from build123d import *

# Parameters (mm, degrees)
F0_R     = 20
F0_R_2   = 2.25
F1_DEPTH = 5
F2_W     = 9.5
F2_H     = 9.5
F2_R     = 2.25
F3_DEPTH = 7
F4_R     = 4.25
F4_R_2   = 2.25
F5_DEPTH = 3


with BuildPart() as f1:
    # F0 (on Top) → F1 (new body)
    with BuildSketch(Plane.XY):
        Circle(F0_R)
        Circle(F0_R_2, mode=Mode.SUBTRACT)
    extrude(amount=F1_DEPTH)

    # F2 (on face) → F3 (join)
    with BuildSketch(Plane.XY.offset(5)):
        Rectangle(F2_W, F2_H)
        Circle(F2_R, mode=Mode.SUBTRACT)
    extrude(amount=F3_DEPTH)

    # F4 (on face) → F5 (cut)
    with BuildSketch(Plane(origin=(0, 0, 0), x_dir=(1, 0, 0), z_dir=(0, 0, -1))):
        Circle(F4_R)
        Circle(F4_R_2, mode=Mode.SUBTRACT)
    extrude(amount=-F5_DEPTH, mode=Mode.SUBTRACT)


solid = f1.part
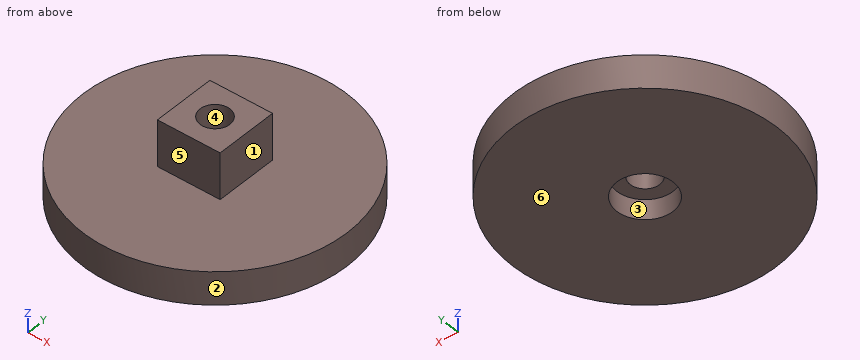
Source: CAD feature listing. Evaluate the final solid. Frame: model axes, mm. Face numbers are marked on the shaded views. A direction names the side the tool comes from. Give positions to 0.01 mm unless a question says otherwise; leave off trailing zeros. Write each loop counter-clockwise with the first axis right and the second up, starting at its lowest first coordinate (ties: lowest second). Pieces come first, ordered by that corner, then holes. Notation, with made-up numbers: M 3,45 L 60,45 A13 ccw 60,70 Z; hole C 22,18.5 d2. An arc over 180 degrees is marked long. Return JSON: item names as keys, results as strings. Group by question number.
1) Draft query along Y for the marked faces 3, 4, 5 and 6. Return one class per face: released by +Y, released by -Y, zero draft, split by the parting line, or undercut.
2) Ray query, L1, parallel to Y at x = 0, z = 7.25; L2, parallel to Y at x = 0, z = 1.6. Return the intervals inside material, ascending.
3) Cut plane D-D, the plane y = -12. Output: boundary loops of the cut face in (x, z), then the cut area to 3 significant figures.
4) Cut plane A-A, the plane y = 0. Output: boundary loops of the cut face in (x, z), then the cut area to 4 significant figures.
5) Cut plane C-C, the plane z = 1. Output: boundary loops of the cut face in (x, y), then the cut area to 3 significant figures.
6) Set-up query: the marked faces 1 and 2. Return all of +Z, -Z, +X, -X, +Y, -Y with unobstructed straight access to the full face (end or side cutting, diameter ignored); none if empty.
7) First-contact query: pin 1 Ø2 at (x, y) = (5.5, 7.5) entering from +Z; pin 2 Ø3.5 at (y, z) = (-0.5, 9.5) entering from +X; pin 3 Ø6 at (x, z) = (0.5, 2.5) entering from -Y; pin 4 Ø10 at (x, y) = (0, 0) entering from -Z. Flat tips, straight axial feed; report the tip coordinate or a pass-through.
Data:
{
 "1": {"face 3": "undercut", "face 4": "undercut", "face 5": "released by -Y", "face 6": "zero draft"},
 "2": {"L1": "y = -4.75 to -2.25, 2.25 to 4.75", "L2": "y = -20 to -4.25, 4.25 to 20"},
 "3": {"outline": "M -16,0 L 16,0 L 16,5 L -16,5 Z", "area": "160 mm²"},
 "4": {"outline": "M -20,0 L -4.25,0 L -4.25,3 L -2.25,3 L -2.25,12 L -4.75,12 L -4.75,5 L -20,5 Z; M 2.25,3 L 4.25,3 L 4.25,0 L 20,0 L 20,5 L 4.75,5 L 4.75,12 L 2.25,12 Z", "area": "200.5 mm²"},
 "5": {"outline": "C 0,0 d40; hole C 0,0 d8.5", "area": "1,200 mm²"},
 "6": {"face 1": "+Z, +X, +Y, -Y", "face 2": "+Z, -Z"},
 "7": {"pin 1": "stops at z = 5", "pin 2": "stops at x = 4.75", "pin 3": "stops at y = -20", "pin 4": "stops at z = 0"}
}
